Work out the finished part from the listing and answer in its coordinate system (mm). A direction names the side the tool comes from. Give positions to 0.01 mm unless a question says otherwise; leave off trailing zeros. Write each loop counter-clockwise with the first axis right and the second up, starting at its lowest first coordinate (ties: lowest second). Pieces come first, ordered by that corner, then holes. Notation, with made-up numbers: (18.5, -17) -> (65.5, -17) arc R24 cw to (65.5, 2) -> close; hole circle Ø6 at (12, 64). An arc over 180 degrees is marked (long way). Write item = value, one per line. Start each with the question number.
from build123d import *

# Parameters (mm, degrees)
SKETCH_1_W               = 35
SKETCH_1_H               = 18.5
EXTRUDE_1_DEPTH          = 3
SKETCH_2_R               = 1.6
SKETCH_2_W               = 23.5
SKETCH_2_H               = 12.5
CUT_EXTRUDE_1_DEPTH      = 40.702015062
SKETCH_3_W               = 2
SKETCH_3_H               = 18.5
EXTRUDE_2_DEPTH          = 3
EXTRUDE_3_DEPTH          = 15
CHAMFER_1_SIZE           = 19.87826233
CHAMFER_1_SIZE_2         = 5.7
SKETCH_6_R               = 1.6
CUT_EXTRUDE_2_DEPTH      = 42.512046444
SKETCH_8_W               = 3
SKETCH_8_H               = 18
EXTRUDE_4_DEPTH          = 8
CHAMFER_2_SIZE           = 3
CUT_EXTRUDE_3_DEPTH      = 46.642633579
CUT_EXTRUDE_3_DEPTH_BACK = 46.642633579
SKETCH_10_R              = 1.6
SKETCH_11_R              = 2.5
CUT_EXTRUDE_4_DEPTH      = 46.642633579
FILLET_1_R               = 3
FILLET_2_R               = 10
CHAMFER_3_SIZE           = 1


with BuildPart() as part:
    # 草图1 → 凸台-拉伸1 (new body)
    with BuildSketch(Plane(origin=(0, 0, 0), x_dir=(1, 0, 0), z_dir=(0, 1, 0))):
        with Locations((17.5, 9.25)):
            Rectangle(SKETCH_1_W, SKETCH_1_H)
    extrude(amount=EXTRUDE_1_DEPTH)

    # 草图2 → 切除-拉伸1 (cut, through all)
    with BuildSketch(Plane(origin=(0, 3, 0), x_dir=(1, 0, 0), z_dir=(0, 1, 0))):
        with Locations(Location((3.75, 9.25, 0), (0, 0, 270))):
            Circle(SKETCH_2_R)
        with Locations(Location((31.25, 9.25, 0), (0, 0, 270))):
            Circle(SKETCH_2_R)
        with Locations((17.5, 9.25)):
            Rectangle(SKETCH_2_W, SKETCH_2_H)
    extrude(amount=-CUT_EXTRUDE_1_DEPTH, mode=Mode.SUBTRACT)

    # 草图3 → 凸台-拉伸2 (add)
    with BuildSketch(Plane(origin=(0, 3, 0), x_dir=(1, 0, 0), z_dir=(0, 1, 0))):
        with Locations((-1, 9.25)):
            Rectangle(SKETCH_3_W, SKETCH_3_H)
    extrude(amount=-EXTRUDE_2_DEPTH)

    # 草图5 → 凸台-拉伸3 (add)
    with BuildSketch(Plane(origin=(0, 0, 0), x_dir=(-1, 0, 0), z_dir=(0, -1, 0))):
        Polygon((-29.25, 15.5), (-1, 15.5), (-1, 3), (-29.25, 3), (-29.25, 0), (2, 0), (2, 3.75), (2, 16.25), (2, 18.5), (-29.25, 18.5), align=None)
    extrude(amount=EXTRUDE_3_DEPTH)

    # 倒角1
    # the kernel refuses this chamfer: 19.87826233, 5.7 mm, written as the material it adds along each edge
    with BuildSketch(Plane(origin=(29.25, 0, -18.5), x_dir=(-0.010616657410321141, -0.9999436417045873, 0), z_dir=(0, 0, 1))) as chamfer_1_piece_1_section:
        Polygon((CHAMFER_1_SIZE * 0.999943641699, CHAMFER_1_SIZE * 0.0106166574103), (-CHAMFER_1_SIZE_2 * 0.0106166574103, CHAMFER_1_SIZE_2 * 0.999943641705), (0, 0), align=None)
    chamfer_1_piece_1 = extrude(amount=3, mode=Mode.PRIVATE)
    chamfer_1_piece_1 = split(chamfer_1_piece_1, bisect_by=Plane(origin=(31.241878904, -15, -17), z_dir=(0, 1, 0)), keep=Keep.TOP, mode=Mode.PRIVATE)
    add(chamfer_1_piece_1)
    with BuildSketch(Plane(origin=(29.25, 0, -70.109385658), x_dir=(-0.010616657410321141, -0.9999436417045873, 0), z_dir=(0, 0, 1))) as chamfer_1_piece_2_section:
        Polygon((CHAMFER_1_SIZE * 0.999943641699, CHAMFER_1_SIZE * 0.0106166574103), (-CHAMFER_1_SIZE_2 * 0.0106166574103, CHAMFER_1_SIZE_2 * 0.999943641705), (0, 0), align=None)
    chamfer_1_piece_2 = extrude(amount=106.218771315, mode=Mode.PRIVATE)
    chamfer_1_piece_2 = split(chamfer_1_piece_2, bisect_by=Plane(origin=(31.241878904, -5.985247808, 0), z_dir=(0, 0, -1)), keep=Keep.TOP, mode=Mode.PRIVATE)
    chamfer_1_piece_2 = split(chamfer_1_piece_2, bisect_by=Plane(origin=(31.241878904, -5.985247808, -3), z_dir=(0, 0, 1)), keep=Keep.TOP, mode=Mode.PRIVATE)
    chamfer_1_piece_2 = split(chamfer_1_piece_2, bisect_by=Plane(origin=(31.241878904, -15, -1.5), z_dir=(0, 1, 0)), keep=Keep.TOP, mode=Mode.PRIVATE)
    add(chamfer_1_piece_2)
    with BuildSketch(Plane(origin=(29.25, 0, -54.609385658), x_dir=(-0.010616657410321141, -0.9999436417045873, 0), z_dir=(0, 0, 1))) as chamfer_1_piece_3_section:
        Polygon((CHAMFER_1_SIZE * 0.999943641699, CHAMFER_1_SIZE * 0.0106166574103), (-CHAMFER_1_SIZE_2 * 0.0106166574103, CHAMFER_1_SIZE_2 * 0.999943641705), (0, 0), align=None)
    chamfer_1_piece_3 = extrude(amount=106.218771315, mode=Mode.PRIVATE)
    chamfer_1_piece_3 = split(chamfer_1_piece_3, bisect_by=Plane(origin=(31.241878904, -5.985247808, -15.5), z_dir=(0, 0, -1)), keep=Keep.TOP, mode=Mode.PRIVATE)
    chamfer_1_piece_3 = split(chamfer_1_piece_3, bisect_by=Plane(origin=(31.241878904, -5.985247808, -18.5), z_dir=(0, 0, 1)), keep=Keep.TOP, mode=Mode.PRIVATE)
    chamfer_1_piece_3 = split(chamfer_1_piece_3, bisect_by=Plane(origin=(31.241878904, -15, -17), z_dir=(0, 1, 0)), keep=Keep.TOP, mode=Mode.PRIVATE)
    add(chamfer_1_piece_3)
    with BuildSketch(Plane(origin=(29.25, 0, -3), x_dir=(-0.010616657410321141, -0.9999436417045873, 0), z_dir=(0, 0, 1))) as chamfer_1_piece_4_section:
        Polygon((CHAMFER_1_SIZE * 0.999943641699, CHAMFER_1_SIZE * 0.0106166574103), (-CHAMFER_1_SIZE_2 * 0.0106166574103, CHAMFER_1_SIZE_2 * 0.999943641705), (0, 0), align=None)
    chamfer_1_piece_4 = extrude(amount=3, mode=Mode.PRIVATE)
    chamfer_1_piece_4 = split(chamfer_1_piece_4, bisect_by=Plane(origin=(31.241878904, -15, -1.5), z_dir=(0, 1, 0)), keep=Keep.TOP, mode=Mode.PRIVATE)
    add(chamfer_1_piece_4)

    # 草图6 → 切除-拉伸2 (cut, through all)
    with BuildSketch(Plane(origin=(1, 0, 0), x_dir=(0, 0, -1), z_dir=(1, 0, 0))):
        with Locations((9.25, -4.6)):
            Circle(SKETCH_6_R)
        with Locations((9.25, -11.4)):
            Circle(SKETCH_6_R)
    extrude(amount=-CUT_EXTRUDE_2_DEPTH, mode=Mode.SUBTRACT)

    # 草图8 → 凸台-拉伸4 (add)
    with BuildSketch(Plane(origin=(0, 0, -18.5), x_dir=(-1, 0, 0), z_dir=(0, 0, -1))):
        with Locations((0.5, -6)):
            Rectangle(SKETCH_8_W, SKETCH_8_H)
    extrude(amount=EXTRUDE_4_DEPTH)

    # 倒角2
    chamfer_2_edges = [part.edges().sort_by_distance(p)[0] for p in [
        (1, -6, -18.5),
    ]]
    chamfer(chamfer_2_edges, length=CHAMFER_2_SIZE)

    # 草图10 → 切除-拉伸3 (cut, two sides: drawn at the far end of the back side and taken through both)
    with BuildSketch(Plane(origin=(1, 0, 0), x_dir=(0, 0, -1), z_dir=(1, 0, 0)).offset(-CUT_EXTRUDE_3_DEPTH_BACK)):
        with Locations((23, -2)):
            Circle(SKETCH_10_R)
        with Locations((23, -10)):
            Circle(SKETCH_10_R)
    extrude(amount=CUT_EXTRUDE_3_DEPTH + CUT_EXTRUDE_3_DEPTH_BACK, mode=Mode.SUBTRACT)

    # 草图11 → 切除-拉伸4 (cut, through all)
    with BuildSketch(Plane(origin=(1, 0, 0), x_dir=(0, 0, -1), z_dir=(1, 0, 0))):
        with Locations((23, -2)):
            Circle(SKETCH_11_R)
        with Locations((23, -10)):
            Circle(SKETCH_11_R)
    extrude(amount=CUT_EXTRUDE_4_DEPTH, mode=Mode.SUBTRACT)

    # 圆角1
    fillet_1_edges = [part.edges().sort_by_distance(p)[0] for p in [
        (-0.5, 3, -26.5),
        (-0.5, -15, -26.5),
    ]]
    fillet(fillet_1_edges, radius=FILLET_1_R)

    # 圆角2
    fillet_2_edges = [part.edges().sort_by_distance(p)[0] for p in [
        (30.648819214, -15, -17),
        (30.648819214, -15, -1.5),
    ]]
    fillet(fillet_2_edges, radius=FILLET_2_R)

    # 倒角3
    chamfer_3_edges = [part.edges().sort_by_distance(p)[0] for p in [
        (1, -7.5, -15.5),
        (1, -7.5, -3),
    ]]
    chamfer(chamfer_3_edges, length=CHAMFER_3_SIZE)


solid = part.part
(1) Determine the mould class of faces 6 (the flat face through (33.822, -3.932, -1.521)), 7 (the cylindrical face through (-0.521, -1.519, -24.526)), 8 (the flat face through (35, 1, -9)) for opening direction Y: pulls with the +Y half, pulls with the -Y half, needs draft (parallel to the pull), parting line crosses it, or undercut.
(2) A cutting plane is placed at B-B, the plane z = -23. Write down the section's boundary in (x, y).
(3) Find the intervals of material crossed by line 1 along X through (y, z) = (1.4, -9.25); line 2 along Y through (x, z) = (-1.25, -23); line 3 along Z through (x, y) = (25, -0.75), in increasing order.
(4) A cutting plane is placed at A-A, the plane z = -5. Write down the section's boundary in (x, y), then the cut area to 3 significant figures.
(5) A cutting plane is placed at C-C, the plane x = 8. Write down the section's boundary in (y, z), then the cut area to 3 significant figures.
(6) For faces 1 (the flat face through (-2, -6, -13)), 2 (the cylindrical face through (-0.48, -10.32, -8.07)), 3 (the flat face through (29.25, 2, -9)), 4 (the flat face through (1.5, -7.4, -15)), 5 (the flat face through (18, -6, -3)), determine the directions among +Z, -Z, +X, -X, +Y, -Y from which every point of the face is accessible in a straight line to the end or side of a thin tool.
(7) A cutting plane is placed at D-D, the plane y = -5.25. Write down the section's boundary in (x, z), then the cut area to 3 significant figures.
(8) Each of these flat-tipped pins is pushed along its axis until it touches: pin 1 (8.5 mm diameter, centred on y = -4.5, z = -11, fed in from +X); pin 2 (5 mm diameter, centred on y = -4.6, z = -9.25, fed in from +X); pin 3 (2 mm diameter, centred on y = -8, z = -17, fed in from +X). Where does it stop, or does it pass through?
Results list:
q1.face_6 = pulls with the -Y half
q1.face_7 = undercut
q1.face_8 = needs draft
q2.outline = (-2, -15) -> (1, -15) -> (1, -11.6) -> (-2, -11.6) -> close; (-2, -8.4) -> (1, -8.4) -> (1, -3.6) -> (-2, -3.6) -> close; (-2, -0.4) -> (1, -0.4) -> (1, 3) -> (-2, 3) -> close
q3.line_1 = -2 to 2.15, 5.35 to 5.75, 29.25 to 29.65, 32.85 to 35
q3.line_2 = -15 to -11.6, -8.4 to -3.6, -0.4 to 3
q3.line_3 = -18.5 to -15.5, -3 to 0
q4.outline = (-2, -15) -> (1, -15) -> (1, 0) -> (5.75, 0) -> (5.75, 3) -> (-2, 3) -> close; (29.25, 0) -> (35, 0) -> (35, 3) -> (29.25, 3) -> close
q4.area = 85.5 mm²
q5.outline = (-15, -18.5) -> (3, -18.5) -> (3, -15.5) -> (-15, -15.5) -> close; (-15, -3) -> (3, -3) -> (3, 0) -> (-15, 0) -> close
q5.area = 108 mm²
q6.face_1 = +Z, -Z, -X, +Y, -Y
q6.face_2 = +X, -X
q6.face_3 = +Y, -Y
q6.face_4 = +X, -Y
q6.face_5 = -Y
q7.outline = (-2, -26.5) -> (1, -26.5) -> (1, -21.5) -> (4, -18.5) -> (33.44, -18.5) -> (33.44, -15.5) -> (2, -15.5) -> (1, -14.5) -> (1, -10.71) -> (-2, -10.71) -> close; (-2, -7.79) -> (1, -7.79) -> (1, -4) -> (2, -3) -> (33.44, -3) -> (33.44, 0) -> (-2, 0) -> close
q7.area = 271 mm²
q8.pin_1 = 1.75
q8.pin_2 = 1
q8.pin_3 = 32.94
